Read the model definition and answer for the solid it produces. Units are mm, in the model's axes. Face numbers are marked on the shaded views. Give positions to 0.01 mm unless a question says otherwise; leave off trailing zeros. Loops run counter-clockwise (first coordinate to the right, second up) from the corner with the lowest first, then second, coordinate; pieces in that order, holes last. Notation, with made-up numbers: (40.5, -20) - (45.5, -20) arc R22 ccw to (45.5, -14) - close; hole circle Ø8 at (-16, 48.25). An arc over 180 degrees is marked (long way). Write item = value, one per line.
```python
from build123d import *

# Parameters (mm, degrees)
EXTRUDE_START       = -2
EXTRUDE_1_DEPTH     = 2
SKETCH_2_R          = 0.6
SKETCH_2_R_2        = 1.25
EXTRUDE_2_DEPTH     = 2
SKETCH_3_R          = 5.9
SKETCH_3_R_2        = 1.25
EXTRUDE_3_DEPTH     = 4
EXTRUDE_4_DEPTH     = 2
SKETCH_5_R          = 1.7
CUT_EXTRUDE_1_DEPTH = 2


# Read off the part's stored shape, not the designer's step: 填料-伸長1
with BuildPart() as part:
    # 填料-伸長1 outline → 填料-伸長1 (new body)
    with BuildSketch(Plane(origin=(0, 18.156954032, 0), x_dir=(1, 0, 0), z_dir=(0, 1, 0)).offset(EXTRUDE_START)):
        with BuildLine():
            Line((-71.976510321, -204.833021781), (-61.351692907, -213.569524655))
            ThreePointArc((-61.351692907, -213.569524655), (-59.430720516, -215.948258819), (-56.577073779, -217.046080048))
            Line((-56.577073779, -217.046080048), (-45.000342303, -224.475246616))
            ThreePointArc((-45.000342303, -224.475246616), (-39.062154339, -223.48095501), (-39.939141491, -217.524312867))
            Line((-39.939141491, -217.524312867), (-50.563958905, -208.787809993))
            ThreePointArc((-50.563958905, -208.787809993), (-52.484931296, -206.409075829), (-55.338578032, -205.3112546))
            Line((-55.338578032, -205.3112546), (-66.915309509, -197.882088033))
            ThreePointArc((-66.915309509, -197.882088033), (-72.853497472, -198.876379638), (-71.976510321, -204.833021781))
        make_face()
        with BuildLine():
            ThreePointArc((-55.939819286, -215.078625755), (-58.253468106, -214.331448143), (-59.674933886, -212.358967399))
            Line((-59.674933886, -212.358967399), (-70.741141251, -203.259521386))
            ThreePointArc((-70.741141251, -203.259521386), (-71.236686796, -200.053632048), (-68.033499603, -199.540910248))
            Line((-68.033499603, -199.540910248), (-55.975832526, -207.278708893))
            ThreePointArc((-55.975832526, -207.278708893), (-53.662183706, -208.025886506), (-52.240717926, -209.998367249))
            Line((-52.240717926, -209.998367249), (-41.17451056, -219.097813262))
            ThreePointArc((-41.17451056, -219.097813262), (-40.678965016, -222.303702601), (-43.882152209, -222.8164244))
            Line((-43.882152209, -222.8164244), (-55.939819286, -215.078625755))
        make_face(mode=Mode.SUBTRACT)
    extrude(amount=EXTRUDE_1_DEPTH)

    # 草圖2 → 填料-伸長2 (add)
    with BuildSketch(Plane(origin=(0, 18.156954032, 0), x_dir=(1, 0, 0), z_dir=(0, 1, 0))):
        with BuildLine():
            Line((-56.577073779, -217.046080048), (-45.000342303, -224.475246616))
            ThreePointArc((-45.000342303, -224.475246616), (-39.06215434, -223.480955011), (-39.939141491, -217.524312867))
            Line((-39.939141491, -217.524312867), (-50.563958905, -208.787809993))
            ThreePointArc((-50.563958905, -208.787809993), (-52.484931296, -206.409075829), (-55.338578032, -205.3112546))
            Line((-55.338578032, -205.3112546), (-66.915309509, -197.882088033))
            ThreePointArc((-66.915309509, -197.882088033), (-72.853497472, -198.876379638), (-71.976510321, -204.833021781))
            Line((-71.976510321, -204.833021781), (-61.351692907, -213.569524655))
            ThreePointArc((-61.351692907, -213.569524655), (-59.430720516, -215.948258819), (-56.577073779, -217.046080048))
        make_face()
        with Locations(Location((-69.943238255, -200.995433976, 0), (0, 0, 180))):
            Circle(SKETCH_2_R, mode=Mode.SUBTRACT)
        with Locations(Location((-68.245587045, -202.231549007, 0), (0, 0, 180))):
            Circle(SKETCH_2_R, mode=Mode.SUBTRACT)
        with Locations(Location((-66.547935835, -203.467664037, 0), (0, 0, 180))):
            Circle(SKETCH_2_R, mode=Mode.SUBTRACT)
        with Locations(Location((-64.850284625, -204.703779068, 0), (0, 0, 180))):
            Circle(SKETCH_2_R, mode=Mode.SUBTRACT)
        with Locations(Location((-63.152633415, -205.939894099, 0), (0, 0, 180))):
            Circle(SKETCH_2_R, mode=Mode.SUBTRACT)
        with Locations(Location((-61.454982205, -207.176009129, 0), (0, 0, 180))):
            Circle(SKETCH_2_R, mode=Mode.SUBTRACT)
        with Locations(Location((-55.957825906, -211.178667324, 0), (0, 0, 180))):
            Circle(SKETCH_2_R_2, mode=Mode.SUBTRACT)
        with Locations(Location((-50.460669607, -215.181325519, 0), (0, 0, 180))):
            Circle(SKETCH_2_R, mode=Mode.SUBTRACT)
        with Locations(Location((-48.763018397, -216.41744055, 0), (0, 0, 180))):
            Circle(SKETCH_2_R, mode=Mode.SUBTRACT)
        with Locations(Location((-47.065367187, -217.65355558, 0), (0, 0, 180))):
            Circle(SKETCH_2_R, mode=Mode.SUBTRACT)
        with Locations(Location((-45.367715977, -218.889670611, 0), (0, 0, 180))):
            Circle(SKETCH_2_R, mode=Mode.SUBTRACT)
        with Locations(Location((-43.670064767, -220.125785642, 0), (0, 0, 180))):
            Circle(SKETCH_2_R, mode=Mode.SUBTRACT)
        with Locations(Location((-41.972413557, -221.361900672, 0), (0, 0, 180))):
            Circle(SKETCH_2_R, mode=Mode.SUBTRACT)
    extrude(amount=EXTRUDE_2_DEPTH)

    # 草圖3 → 填料-伸長3 (add)
    with BuildSketch(Plane(origin=(0, 20.156954032, 0), x_dir=(1, 0, 0), z_dir=(0, 1, 0))):
        with Locations(Location((-55.957825906, -211.178667324, 0), (0, 0, 180))):
            Circle(SKETCH_3_R)
        with Locations(Location((-55.957825906, -211.178667324, 0), (0, 0, 180))):
            Circle(SKETCH_3_R_2, mode=Mode.SUBTRACT)
    extrude(amount=EXTRUDE_3_DEPTH)

    # 草圖4 → 填料-伸長4 (add)
    with BuildSketch(Plane(origin=(0, 24.156954032, 0), x_dir=(1, 0, 0), z_dir=(0, 1, 0))):
        Polygon((-61.351692907, -213.569524655), (-55.338578032, -205.3112546), (-99.800871628, -172.93681332), (-105.813986502, -181.195083375), align=None)
    extrude(amount=-EXTRUDE_4_DEPTH)

    # 草圖5 → 除料-伸長1 (cut)
    with BuildSketch(Plane.XZ.offset(-22.156954032)):
        with Locations((-76.167959358, 196.463012197)):
            Circle(SKETCH_5_R)
    extrude(amount=-CUT_EXTRUDE_1_DEPTH, mode=Mode.SUBTRACT)


solid = part.part
```
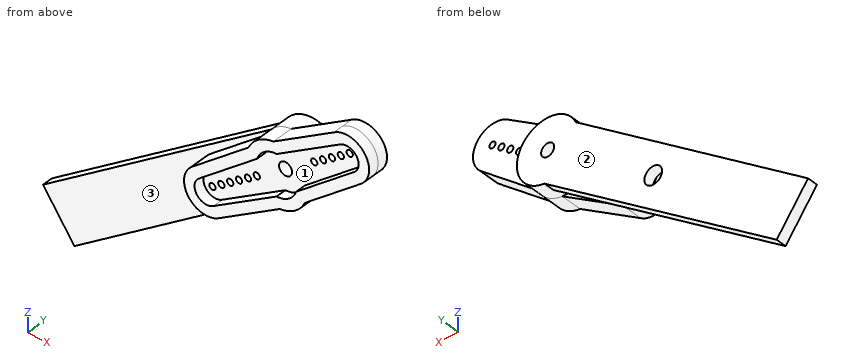
1) A cutting plane is placed at B-B on x = -77. Determine the outline of the cut face in (y, z), then the cut area to 3 significant figures.
Output:
outline = (22.16, 189.54) - (24.16, 189.54) - (24.16, 194.98) - (22.16, 194.98) - close; (22.16, 197.95) - (24.16, 197.95) - (24.16, 202.18) - (22.16, 202.18) - close
area = 19.3 mm²
2) Find the intervals of material crossed by probe 1 along Y at (x, z) = (-63, 211); probe 2 along Y at (x, z) = (-44, 221); probe 3 along Z at (x, y) = (-41.5, 19), in increasing order.
Output:
probe_1 = 16.16 to 20.16, 22.16 to 24.16
probe_2 = 18.16 to 20.16
probe_3 = 216.24 to 220.99, 221.73 to 225.12
3) A cutting plane is placed at D-D on x = -87. Determine the outline of the cut face in (y, z), then the cut area to 3 significant figures.
Output:
outline = (22.16, 182.26) - (24.16, 182.26) - (24.16, 194.89) - (22.16, 194.89) - close
area = 25.3 mm²
4) The mould has two halves that part along Y. Classify the marked faces 1, 2 and 3: pulls with the +Y half, pulls with the -Y half, needs draft (parallel to the pull), parting line crosses it, or undercut.
Output:
face_1 = pulls with the -Y half
face_2 = pulls with the +Y half
face_3 = undercut
5) Each of these flat-tipped pins is pushed along its axis until it touches: P1, Ø1.9, axis at x = -61.45, z = 207.18, coming from the -Y side; P2, Ø2, axis at x = -55.5, y = 19.5, coming from the +Z side; P3, Ø12, axis at x = -70, z = 189.5, coming from the -Y side; P4, Ø1.1, axis at x = -45.37, z = 218.89, coming from the +Y side. Where does it stop, or does it pass through?
Output:
P1 = 18.16
P2 = 218.38
P3 = 22.16
P4 = through
6) A cutting plane is placed at C-C on z = 183.5. Determine the outline of the cut face in (x, y), then the cut area to 3 significant figures.
Output:
outline = (-102.65, 22.16) - (-85.29, 22.16) - (-85.29, 24.16) - (-102.65, 24.16) - close
area = 34.7 mm²
7) A cutting plane is placed at A-A on y = 17. Determine the outline of the cut face in (x, z), then the cut area to 3 significant figures.
Output:
outline = (-71.98, 204.83) arc R4.3 ccw to (-66.92, 197.88) - (-55.34, 205.31) arc R5.9 ccw to (-50.56, 208.79) - (-39.94, 217.52) arc R4.3 ccw to (-45, 224.48) - (-56.58, 217.05) arc R5.9 ccw to (-61.35, 213.57) - close; hole (-70.74, 203.26) arc R2.3 ccw to (-68.03, 199.54) - (-55.98, 207.28) arc R3.9 ccw to (-52.24, 210) - (-41.17, 219.1) arc R2.3 ccw to (-43.88, 222.82) - (-55.94, 215.08) arc R3.9 ccw to (-59.67, 212.36) - close
area = 176 mm²
